Design review of the part built by this model. Coordinates are the model's own, in mm. Face numbers are marked on the shaded views. A direction names the side the tool comes from. Round coordinates to 2 decimals unless told otherwise and drop trailing zeros. Loops run counter-clockwise (first coordinate to the right, second up) from the corner with the lowest first, then second, coordinate; pieces in that order, holes last. Notation, with made-up numbers: M 3,-15 L 42,-15 A21 cw 42,-2 Z; hole C 79,43.5 d6. An arc over 180 degrees is marked long. One line per item, written item: value. Start each with the question number.
Item 1: We need section B-B (y = 0). Write out the cut boundary in (x, z), then the cut area to 3 significant figures.
Item 2: For line 1 along Y through (x, z) = (-4.5, -0.75); line 2 along Y through (x, z) = (22.5, -4); line 3 along X through (y, z) = (15, -4.5), list the stretches that pass through material, from the lowest coordinate up.
Item 3: Mouldability with a two-part tool opening along Y and no side actions: class the marked faces 1, 2, 3 and 4 as released by +Y, released by -Y, zero draft, split by the parting line, or undercut.
Item 4: We need section A-A (z = -2.25). State how many separate pieces and enclosed holes the cut face has, then the cut area to 3 significant figures.
Item 5: For the marked faces 5 and 6, list the 3-axis set-ups (+Z, -Z, +X, -X, +Y, -Y) from which the entire face can be reached by the end or side of a thin tool; tool diameter is ignored.
Item 6: We need section D-D (y = -9). Write out the cut boundary in (x, z), then the cut area to 3 significant figures.
Item 7: Clearance check with flat-ended pins moving along their axes: pin 1 (6 mm diameter, centred on x = 2, y = 0, fed in from -Z); pin 2 (0.6 mm diameter, centred on x = -22.5, y = 0, fed in from -Z). State where each tip first meets the part, or that it passes through.
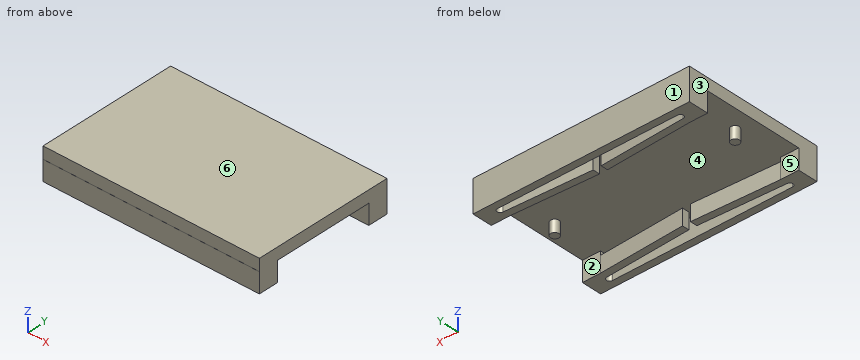
from build123d import *

# Parameters (mm, degrees)
SKETCH1_R             = 1.05
BOSS_EXTRUDE1_DEPTH   = 3
BOSS_EXTRUDE1_2_DEPTH = 3
SKETCH1_3_W           = 54
SKETCH1_3_H           = 24.978925024
BOSS_EXTRUDE2_DEPTH   = 3
BOSS_EXTRUDE4_START   = -3
SKETCH4_W             = 54
SKETCH4_H             = 5
BOSS_EXTRUDE4_DEPTH   = 3
BOSS_EXTRUDE5_DEPTH   = 5
BOSS_EXTRUDE6_DEPTH   = 5
SKETCH6_W             = 45
SKETCH6_H             = 1
CUT_EXTRUDE1_DEPTH    = 2.5
SKETCH7_W             = 45
SKETCH7_H             = 1
CUT_EXTRUDE2_DEPTH    = 2.5


with BuildPart() as part:
    # Sketch1 → Boss-Extrude1 (new body)
    with BuildSketch(Plane.XY):
        with Locations((-22.5, 0)):
            Circle(SKETCH1_R)
    extrude(amount=-BOSS_EXTRUDE1_DEPTH)



with BuildPart() as body_2:
    # Sketch1 → Boss-Extrude1 2 (new body)
    with BuildSketch(Plane.XY):
        with Locations((22.5, 0)):
            Circle(SKETCH1_R)
    extrude(amount=-BOSS_EXTRUDE1_2_DEPTH)


with BuildPart() as part_1:
    add(part.part)

    add(body_2.part)  # Boss-Extrude2 merges body 2
    # Sketch1<3> → Boss-Extrude2 (add)
    with BuildSketch(Plane.XY):
        with Locations((0, -0.010537488)):
            Rectangle(SKETCH1_3_W, SKETCH1_3_H)
    extrude(amount=BOSS_EXTRUDE2_DEPTH)

    # Sketch4 → Boss-Extrude4 (add)
    with BuildSketch(Plane.XY.offset(3).offset(BOSS_EXTRUDE4_START)):
        with Locations((0, 14.978925024)):
            Rectangle(SKETCH4_W, SKETCH4_H)
        with Locations((0, -14.978925024)):
            Rectangle(SKETCH4_W, SKETCH4_H)
    extrude(amount=BOSS_EXTRUDE4_DEPTH)

    # Sketch3 → Boss-Extrude5 (add)
    with BuildSketch(Plane(origin=(0, 0, 0), x_dir=(-1, 0, 0), z_dir=(0, 0, -1))):
        with BuildLine():
            Line((-27, 12.478925024), (-22.5, 12.478925024))
            Line((-22.5, 12.478925024), (-1, 11.35215777))
            Line((-1, 11.35215777), (-1, 13.104559375))
            Line((-1, 13.104559375), (-22.5, 14.23132663))
            ThreePointArc((-22.5, 14.23132663), (-23.25, 14.98132663), (-22.5, 15.73132663))
            Line((-22.5, 15.73132663), (22.5, 15.73132663))
            ThreePointArc((22.5, 15.73132663), (23.25, 14.98132663), (22.5, 14.23132663))
            Line((22.5, 14.23132663), (1, 13.104559375))
            Line((1, 13.104559375), (1, 11.35215777))
            Line((1, 11.35215777), (22.5, 12.478925024))
            Line((22.5, 12.478925024), (27, 12.478925024))
            Line((27, 12.478925024), (27, 17.478925024))
            Line((27, 17.478925024), (-27, 17.478925024))
            Line((-27, 17.478925024), (-27, 12.478925024))
        make_face()
    extrude(amount=BOSS_EXTRUDE5_DEPTH)

    # Sketch3<4> → Boss-Extrude6 (add)
    with BuildSketch(Plane(origin=(0, 0, 0), x_dir=(-1, 0, 0), z_dir=(0, 0, -1))):
        with BuildLine():
            Line((1, -13.125634351), (1, -11.373232745))
            Line((1, -11.373232745), (22.5, -12.5))
            Line((22.5, -12.5), (27, -12.5))
            Line((27, -12.5), (27, -17.5))
            Line((27, -17.5), (-27, -17.5))
            Line((-27, -17.5), (-27, -12.5))
            Line((-27, -12.5), (-22.5, -12.5))
            Line((-22.5, -12.5), (-1, -11.373232745))
            Line((-1, -11.373232745), (-1, -13.125634351))
            Line((-1, -13.125634351), (-22.5, -14.252401605))
            ThreePointArc((-22.5, -14.252401605), (-23.25, -15.002401605), (-22.5, -15.752401605))
            Line((-22.5, -15.752401605), (22.5, -15.752401605))
            ThreePointArc((22.5, -15.752401605), (23.25, -15.002401605), (22.5, -14.252401605))
            Line((22.5, -14.252401605), (1, -13.125634351))
        make_face()
    extrude(amount=BOSS_EXTRUDE6_DEPTH)

    # Sketch6 → Cut-Extrude1 (cut, symmetric)
    with BuildSketch(Plane.XZ.offset(-12.478925024)):
        with Locations((0, -0.5)):
            Rectangle(SKETCH6_W, SKETCH6_H)
    extrude(amount=CUT_EXTRUDE1_DEPTH, both=True, mode=Mode.SUBTRACT)

    # Sketch7 → Cut-Extrude2 (cut, symmetric)
    with BuildSketch(Plane(origin=(0, -12.5, 0), x_dir=(1, 0, 0), z_dir=(0, 1, 0))):
        with Locations((0, 0.5)):
            Rectangle(SKETCH7_W, SKETCH7_H)
    extrude(amount=CUT_EXTRUDE2_DEPTH, both=True, mode=Mode.SUBTRACT)


solid = part_1.part
A:
1. outline: M -27,0 L -23.55,0 L -23.55,-3 L -21.45,-3 L -21.45,0 L 21.45,0 L 21.45,-3 L 23.55,-3 L 23.55,0 L 27,0 L 27,3 L -27,3 Z
1. area: 175 mm2
2. line 1: -17.5 to -15.75, 15.73 to 17.48
2. line 2: -17.5 to -15.75, -14.25 to -12.5, 12.48 to 14.23, 15.73 to 17.48
2. line 3: -27 to -23.25, 23.25 to 27
3. face 1: released by +Y
3. face 2: undercut
3. face 3: zero draft
3. face 4: undercut
4. separate pieces: 4
4. enclosed holes: 0
4. area: 401 mm2
5. face 5: -Z, -X
5. face 6: +Z, +X, -X, +Y, -Y
6. outline: M -27,0 L 27,0 L 27,3 L -27,3 Z
6. area: 162 mm2
7. pin 1: z = 0
7. pin 2: z = -3
